Geometry check sheet. Reference: the model listing, model coordinates, mm. Round coordinates to 2 decimals unless told otherwise and drop trailing zeros. Write each loop counter-clockwise with the first axis right and the second up, starting at its lowest first coordinate (ties: lowest second). Pieces come first, ordered by that corner, then holes. Notation, with made-up numbers: M -40,86.25 L -27,86.25 A25 cw -27,107.25 Z; hole C 8,53 d3. An arc over 180 degrees is marked long. Put each result on its own line as item: value. Start each with the question number.
(1) Mould release check, pull along X, two halves, no side actions. Record for faces 1 (the flat face through (2, -758, -5.868)), 2 (the flat face through (2, -758, -2.693)): pulls with the +X half, pulls with the -X half, needs draft (parallel to the pull), parting line crosses it, or undercut.
(2) Material ranges on probe 1 along Y at (x, z) = (0.5, -4.5); probe 2 along X at (y, z) = (-695, -6.25); probe 3 along Y at (x, z) = (-1, -4.25), recorded low to high.
(3) Section check B-B on y = -846.5. Record the cut outline in (x, z).
(4) Section check A-A on z = -11.5. Record the cut outline in (x, y).
(5) Gauge pin test, flat ends, axial feed: pin 1 (4 mm diameter, centred on x = -8, y = -773, fed in from -Z); pin 2 (9 mm diameter, centred on x = 1.74, y = -28.58, fed in from -Z) (3 decimals). Record the tip position at first contact, or that the pin passes through.
from build123d import *

# Parameters (mm, degrees)
F1_DEPTH = 1536.7
F2_R     = 5
F3_DEPTH = 25.4


with BuildPart() as f1:
    # F0 (on Front) → F1 (new body)
    with BuildSketch(Plane.XZ):
        Polygon((17.614564, -2.693408), (-14.135436, -2.693408), (-14.135436, -15.393408), (-10.960436, -15.393408), (-10.960436, -5.868408), (14.439564, -5.868408), (14.439564, -15.393408), (17.614564, -15.393408), align=None)
    extrude(amount=F1_DEPTH)

    # F2 (on face) → F3 (cut)
    with BuildSketch(Plane.XY.offset(-2.693408)):
        with Locations((1.739564, -1508.125)):
            Circle(F2_R)
        with Locations((1.739564, -28.575)):
            Circle(F2_R)
    extrude(amount=-F3_DEPTH, mode=Mode.SUBTRACT)


solid = f1.part
Answers follow:
1. face 1: undercut
1. face 2: needs draft
2. probe 1: y = -1536.7 to -1512.97, -1503.28 to -33.42, -23.73 to 0
2. probe 2: x = -14.14 to -10.96, 14.44 to 17.61
2. probe 3: y = -1536.7 to -1512.31, -1503.94 to -32.76, -24.39 to 0
3. outline: M -14.14,-15.39 L -10.96,-15.39 L -10.96,-5.87 L 14.44,-5.87 L 14.44,-15.39 L 17.61,-15.39 L 17.61,-2.69 L -14.14,-2.69 Z
4. outline: M -14.14,-1536.7 L -10.96,-1536.7 L -10.96,0 L -14.14,0 Z; M 14.44,-1536.7 L 17.61,-1536.7 L 17.61,0 L 14.44,0 Z
5. pin 1: stops at z = -5.87
5. pin 2: passes through
